Source: CAD feature listing. Evaluate the final solid. Frame: model axes, mm. A direction names the side the tool comes from. Round coordinates to 2 decimals unless told otherwise and drop trailing zeros. Order: outer loops, then holes, each group sorted by start corner. A loop starts at its lowest first (then second) coordinate and runs counter-clockwise, first axis right, second up. Notation, with made-up numbers: M 31,8.25 L 78,8.25 A23 cw 78,36.25 Z; hole C 74,-38 d10. An arc over 180 degrees is marked long. Use CSV: the item, a comma, the result in double quotes. Start each with the question number.
```python
from build123d import *

# Parameters (mm, degrees)
SKETCH1_R           = 200
BOSS_EXTRUDE1_DEPTH = 10
SKETCH2_R           = 6.25
CUT_EXTRUDE1_DEPTH  = 284.019433962
SKETCH3_R           = 35
CUT_EXTRUDE2_DEPTH  = 284.019433962
SKETCH4_R           = 3.05
CUT_EXTRUDE3_DEPTH  = 284.019433962
CIRPATTERN1_COUNT   = 8
SKETCH5_R           = 2.05
CUT_EXTRUDE4_DEPTH  = 284.019433962
CIRPATTERN2_COUNT   = 4
CUT_EXTRUDE5_START  = -10
CUT_EXTRUDE5_DEPTH  = 10
CIRPATTERN3_COUNT   = 4
FILLET1_R           = 10
CUT_EXTRUDE6_DEPTH  = 282.602556807


with BuildPart() as part:
    # Sketch1 → Boss-Extrude1 (new body)
    with BuildSketch(Plane(origin=(0, 0, 0), x_dir=(1, 0, 0), z_dir=(0, 1, 0))):
        with Locations(Location((0, 0, 0), (0, 0, 270))):
            Circle(SKETCH1_R)
    extrude(amount=BOSS_EXTRUDE1_DEPTH)

    # Sketch2 → Cut-Extrude1 (cut, through all)
    with BuildSketch(Plane(origin=(0, 10, 0), x_dir=(1, 0, 0), z_dir=(0, 1, 0))):
        with Locations(Location((-135.764501988, 0, 0), (0, 0, 270))):
            Circle(SKETCH2_R)
        with Locations(Location((0, -135.764501988, 0), (0, 0, 270))):
            Circle(SKETCH2_R)
        with Locations(Location((135.764501988, 0, 0), (0, 0, 270))):
            Circle(SKETCH2_R)
        with Locations(Location((0, 135.764501988, 0), (0, 0, 270))):
            Circle(SKETCH2_R)
    extrude(amount=-CUT_EXTRUDE1_DEPTH, mode=Mode.SUBTRACT)

    # Sketch3 → Cut-Extrude2 (cut, through all)
    with BuildSketch(Plane(origin=(0, 10, 0), x_dir=(1, 0, 0), z_dir=(0, 1, 0))):
        with Locations(Location((0, 0, 0), (0, 0, 270))):
            Circle(SKETCH3_R)
    extrude(amount=-CUT_EXTRUDE2_DEPTH, mode=Mode.SUBTRACT)

    # Sketch4 → Cut-Extrude3 (cut, through all)
    with BuildSketch(Plane(origin=(0, 10, 0), x_dir=(1, 0, 0), z_dir=(0, 1, 0))):
        with Locations(Location((17.220754456, 41.574578963, 0), (0, 0, 270))):
            Circle(SKETCH4_R)
    cut_extrude3 = extrude(amount=-CUT_EXTRUDE3_DEPTH, mode=Mode.SUBTRACT)

    # CirPattern1: Cut-Extrude3 ×8 about axis
    cirpattern1_axis = Axis((0, 0, 0), (0, 1, 0))
    for i in range(1, CIRPATTERN1_COUNT):
        add(cut_extrude3.rotate(cirpattern1_axis, i * 360 / CIRPATTERN1_COUNT), mode=Mode.SUBTRACT)

    # Sketch5 → Cut-Extrude4 (cut, through all)
    with BuildSketch(Plane(origin=(0, 10, 0), x_dir=(1, 0, 0), z_dir=(0, 1, 0))):
        with Locations(Location((-188.264501988, 8.25, 0), (0, 0, 270))):
            Circle(SKETCH5_R)
        with Locations(Location((-174.764501988, 8.25, 0), (0, 0, 270))):
            Circle(SKETCH5_R)
        with Locations(Location((-174.764501988, -8.25, 0), (0, 0, 270))):
            Circle(SKETCH5_R)
        with Locations(Location((-188.264501988, -8.25, 0), (0, 0, 270))):
            Circle(SKETCH5_R)
    cut_extrude4 = extrude(amount=-CUT_EXTRUDE4_DEPTH, mode=Mode.SUBTRACT)

    # CirPattern2: Cut-Extrude4 ×4 about axis
    cirpattern2_axis = Axis((0, 0, 0), (0, 1, 0))
    for i in range(1, CIRPATTERN2_COUNT):
        add(cut_extrude4.rotate(cirpattern2_axis, i * 360 / CIRPATTERN2_COUNT), mode=Mode.SUBTRACT)

    # Sketch6 → Cut-Extrude5 (cut)
    with BuildSketch(Plane(origin=(0, 10, 0), x_dir=(1, 0, 0), z_dir=(0, 1, 0)).offset(CUT_EXTRUDE5_START)):
        with BuildLine():
            Line((-198.997487421, 20), (-118.321595662, 20))
            ThreePointArc((-118.321595662, 20), (-84.852813742, 84.852813742), (-20, 118.321595662))
            Line((-20, 118.321595662), (-20, 198.997487421))
            ThreePointArc((-20, 198.997487421), (-141.421356237, 141.421356237), (-198.997487421, 20))
        make_face()
        with BuildLine():
            Line((-198.997487421, -20), (-198.997487421, 20))
            ThreePointArc((-198.997487421, 20), (-200, 0), (-198.997487421, -20))
        make_face()
    cut_extrude5 = extrude(amount=CUT_EXTRUDE5_DEPTH, mode=Mode.SUBTRACT)

    # CirPattern3: Cut-Extrude5 ×4 about axis
    cirpattern3_axis = Axis((0, 0, 0), (0, 1, 0))
    for i in range(1, CIRPATTERN3_COUNT):
        add(cut_extrude5.rotate(cirpattern3_axis, i * 360 / CIRPATTERN3_COUNT), mode=Mode.SUBTRACT)

    # Fillet1
    fillet1_edges = [part.edges().sort_by_distance(p)[0] for p in [
        (-198.997487421, 5, -20),
        (-20, 5, -198.997487421),
        (-198.997487421, 5, 20),
        (20, 5, -198.997487421),
        (198.997487421, 5, -20),
        (198.997487421, 5, 20),
        (20, 5, 198.997487421),
        (-20, 5, 198.997487421),
    ]]
    fillet(fillet1_edges, radius=FILLET1_R)

    # Sketch7 → Cut-Extrude6 (cut, through all)
    with BuildSketch(Plane(origin=(0, 10, 0), x_dir=(1, 0, 0), z_dir=(0, 1, 0))):
        Polygon((77.781745931, 77.781745931), (68.122487668, 75.193555479), (75.193555479, 68.122487668), align=None)
    extrude(amount=-CUT_EXTRUDE6_DEPTH, mode=Mode.SUBTRACT)


solid = part.part
```
(1) Line query: line 1 along X through (y, z) = (8, 175); line 2 along Z through (x, y) = (-8.25, 6.5); line 3 along X through (y, z) = (9.5, -39.5) (3 decimals). Output: solid intervals per line, ascending.
(2) Section A-A on z = 0. Return loops of the section in (x, y).
(3) Section B-B on x = 0. Return loops of the section in (y, z).
(4) Reachability of faces 5 (the face through (154, 5, 20)), 6 (the face through (-153, 5, 20)), 7 (the face through (153, 5, -20)) from +Z, -Z, +X, -X, +Y, -Y: full face, straight path, thin tool, end or side. Return the list, or none.
(5) Section C-C on y = 6.75. Give the number of separate pieces and of enclosed holes in the cut face, plus the area to 3 significant figures.
(6) Contact query for flat-ended pins moving along their axis: P1, Ø5, axis at x = 160.5, y = 7, coming from the +Z side; P2, Ø5, axis at x = 164, y = 4, coming from the -Z side; P3, Ø14.5, axis at x = 135.76, z = 0, coming from the +Y side; P4, Ø1, axis at y = 8.5, z = -81, coming from the -X side. Output: stop coordinate, or through.
(7) Draft query along Z for faces 1 (the face through (73, 5.1, -76.5)), 2 (the face through (20, 5, 153)), 3 (the face through (-21, 5, -28)), 4 (the face through (-17.15, 5.07, -195.99)). Return one class per face: pulls with the +Z half, pulls with the -Z half, needs draft (parallel to the pull), parting line crosses it, or undercut.
(8) Section D-D on z = -149.5. Return loops of the section in (x, y), plus the area to 3 significant figures.
Results below:
1,line 1,"x = -20 to -10.29, -6.21 to 6.21, 10.29 to 20"
1,line 2,"z = -199 to -190.31, -186.21 to -176.81, -172.71 to -34.01, 34.01 to 172.71, 176.81 to 186.21, 190.31 to 199"
1,line 3,"x = -113.313 to -19.457, -14.985 to 14.985, 19.457 to 113.313"
2,outline,"M -199,0 L -142.01,0 L -142.01,10 L -199,10 Z; M -129.51,0 L -35,0 L -35,10 L -129.51,10 Z; M 35,0 L 129.51,0 L 129.51,10 L 35,10 Z; M 142.01,0 L 199,0 L 199,10 L 142.01,10 Z"
3,outline,"M 0,-199 L 10,-199 L 10,-142.01 L 0,-142.01 Z; M 0,-129.51 L 10,-129.51 L 10,-35 L 0,-35 Z; M 0,35 L 10,35 L 10,129.51 L 0,129.51 Z; M 0,142.01 L 10,142.01 L 10,199 L 0,199 Z"
4,face 5,"+Z, +X, +Y, -Y"
4,face 6,"+Z, -X, +Y, -Y"
4,face 7,"-Z, +X, +Y, -Y"
5,separate pieces,"1"
5,enclosed holes,"30"
5,area,"53,000 mm2"
6,P1,"stops at z = 20"
6,P2,"stops at z = -20"
6,P3,"stops at y = 10"
6,P4,"stops at x = -88.99"
7,face 1,"undercut"
7,face 2,"needs draft"
7,face 3,"undercut"
7,face 4,"pulls with the -Z half"
8,outline,"M -20,0 L 20,0 L 20,10 L -20,10 Z"
8,area,"400 mm2"
